from build123d import *

# Parameters (mm, degrees)
SKETCH1_R                 = 10
BOSS_EXTRUDE1_DEPTH       = 20
CUT_EXTRUDE1_DEPTH        = 103
M8X1_0_TAPPED_HOLE1_D     = 7
M8X1_0_TAPPED_HOLE1_DEPTH = 19
M8X1_0_TAPPED_HOLE1_TIP   = 2.103012167


with BuildPart() as part:
    # Sketch1 → Boss-Extrude1 (new body)
    with BuildSketch(Plane.XY):
        Circle(SKETCH1_R)
    extrude(amount=BOSS_EXTRUDE1_DEPTH)

    # Sketch2 → Cut-Extrude1 (cut, symmetric)
    with BuildSketch(Plane(origin=(0, 0, 0), x_dir=(1, 0, 0), z_dir=(0, 1, 0))):
        Polygon((-175.190419067, 2.685826336), (24.809580933, -21.814173664), (24.809580933, -148.814173664), (-175.190419067, -173.314173664), align=None)
    extrude(amount=CUT_EXTRUDE1_DEPTH, both=True, mode=Mode.SUBTRACT)

    # M8x1.0 Tapped Hole1
    with Locations(Plane(origin=(0, 0, 0), x_dir=(-1, 0, 0), z_dir=(0, 0, -1))):
        with Locations((0, 0)):
            Hole(M8X1_0_TAPPED_HOLE1_D / 2, depth=M8X1_0_TAPPED_HOLE1_DEPTH)
            with Locations((0, 0, -(M8X1_0_TAPPED_HOLE1_DEPTH + M8X1_0_TAPPED_HOLE1_TIP / 2))):  # 118° drill point
                Cone(0, M8X1_0_TAPPED_HOLE1_D / 2, M8X1_0_TAPPED_HOLE1_TIP, mode=Mode.SUBTRACT)


solid = part.part
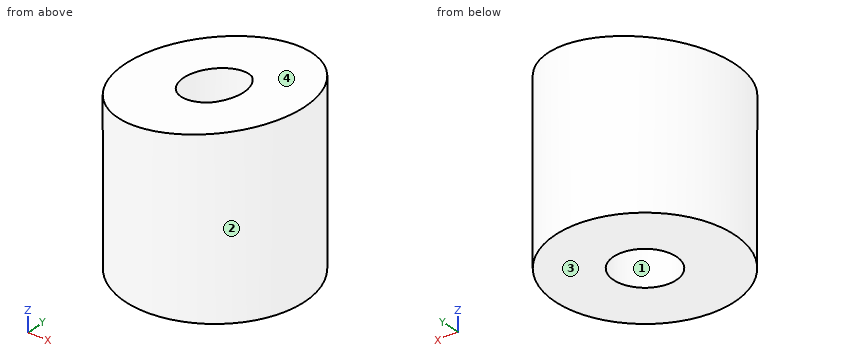
For this review, take the finished solid that the model builds, in its own axes (mm). Face numbers are marked on the shaded views. Give positions to 0.01 mm unless a question says otherwise; leave off trailing zeros. Order: outer loops, then holes, each group sorted by start corner. A loop starts at its lowest first (then second) coordinate and runs counter-clockwise, first axis right, second up. Notation, with made-up numbers: (65, 32) - (102, 32) arc R32 cw to (102, 65) - close; hole circle Ø3 at (17.5, 48.5). An arc over 180 degrees is marked (long way). Answer as a JSON object with one key per item and string values. Group by question number.
Item 1: Take a section at D-D on x = 6. Give the boundary of the cut face in (y, z), and give its area (3 significant figures).
Item 2: Take a section at B-B on y = 0. Give the boundary of the cut face in (x, z).
Item 3: Wall thickness on line 1 along X through (y, z) = (0, 10); line 2 along Y through (x, z) = (1.25, 10): over which ranges is each line inside the solid? List them lowest first.
Item 4: Take a section at A-A on x = 0. Give the boundary of the cut face in (y, z) (3 decimals), and give its area (3 significant figures).
Item 5: Draft analysis for pull direction X (two halves, no side actions). For the marked faces 1, 2, 3 and 4, state which applies: pulls with the +X half, pulls with the -X half, needs draft (parallel to the pull), parting line crosses it, or undercut.
Item 6: Clearance check with flat-ended pins moving along their axes: pin 1 Ø2 at (x, z) = (-5.5, 3.5) entering from +Y; pin 2 Ø2 at (x, y) = (4.5, 5) entering from +Z; pin 3 Ø1 at (x, z) = (1, 15) entering from -Y. State where each tip first meets the part, or that it passes through.
Item 7: Take a section at C-C on z = 7.5. Give the boundary of the cut face in (x, y), and give its area (3 significant figures).
Reported:
{
 "1": {"outline": "(-8, 0) - (8, 0) - (8, 19.51) - (-8, 19.51) - close", "area": "312 mm^2"},
 "2": {"outline": "(-10, 0) - (-3.5, 0) - (-3.5, 18.35) - (-10, 17.55) - close; (3.22, 19.17) - (3.5, 19) - (3.5, 0) - (10, 0) - (10, 20) - close"},
 "3": {"line 1": "-10 to -3.5, 3.5 to 10", "line 2": "-9.92 to -3.27, 3.27 to 9.92"},
 "4": {"outline": "(-10, 0) - (-3.5, 0) - (-3.5, 18.775) - (-10, 18.775) - close; (3.5, 0) - (10, 0) - (10, 18.775) - (3.5, 18.775) - close", "area": "244 mm^2"},
 "5": {"face 1": "undercut", "face 2": "parting line crosses it", "face 3": "needs draft", "face 4": "pulls with the -X half"},
 "6": {"pin 1": "y = 8.93", "pin 2": "z = 19.45", "pin 3": "y = -9.99"},
 "7": {"outline": "circle Ø20 at (0, 0); hole circle Ø7 at (0, 0)", "area": "276 mm^2"}
}
